```python
from build123d import *

# Parameters (mm, degrees)
VARREDURA_FINO1_PROFILE_R   = 6
VARREDURA_FINO1_PROFILE_R_2 = 5
RESSALTO_EXTRUS_O1_DEPTH    = 1


with BuildPart() as part:
    # Varredura-Fino1: sweep along a path in Esbo_o1
    with BuildLine(Plane.XY) as varredura_fino1_path:
        Line((0, -13.453624047), (-6.689647316, -7.432941462))
        ThreePointArc((-6.689647316, -7.432941462), (-9.74420246, 2.247335849), (-2.758518872, 9.612001541))
        Line((-2.758518872, 9.612001541), (13.460564792, 14.266666669))
    # Varredura-Fino1 profile (on start of the path) → Varredura-Fino1 (sweep)
    with BuildSketch(Plane(origin=(0, -13.453624047, 0), x_dir=(-0.6689647316224496, -0.7432941462471664, 0), z_dir=(-0.7432941462471664, 0.6689647316224496, 0))):
        Circle(VARREDURA_FINO1_PROFILE_R)
        Circle(VARREDURA_FINO1_PROFILE_R_2, mode=Mode.SUBTRACT)
    sweep(path=varredura_fino1_path.line)

    # Esbo_o19 → Ressalto-extrus_o1 (add)
    with BuildSketch(Plane(origin=(0, 0, -6), x_dir=(-1, 0, 0), z_dir=(0, 0, -1))):
        with BuildLine():
            Line((-13.046786961, 15.7084669), (-12.770935074, 16.669667054))
            Line((-12.770935074, 16.669667054), (-19.499336153, 18.600630265))
            ThreePointArc((-19.499336153, 18.600630265), (-22.591966256, 16.887259598), (-20.878595589, 13.794629494))
            Line((-20.878595589, 13.794629494), (-14.15019451, 11.863666283))
            Line((-14.15019451, 11.863666283), (-13.874342623, 12.824866438))
            Line((-13.874342623, 12.824866438), (-20.602743702, 14.755829648))
            ThreePointArc((-20.602743702, 14.755829648), (-21.630766102, 16.61140771), (-19.77518804, 17.639430111))
            Line((-19.77518804, 17.639430111), (-13.046786961, 15.7084669))
        make_face()
        with BuildLine():
            Line((-2.006894195, -11.223741608), (-2.675858926, -10.480447462))
            Line((-2.675858926, -10.480447462), (-7.87891795, -15.163200583))
            ThreePointArc((-7.87891795, -15.163200583), (-8.176235609, -20.812236095), (-2.527200097, -21.109553753))
            Line((-2.527200097, -21.109553753), (2.675858926, -16.426800632))
            Line((2.675858926, -16.426800632), (2.006894195, -15.683506486))
            Line((2.006894195, -15.683506486), (-3.196164829, -20.366259607))
            ThreePointArc((-3.196164829, -20.366259607), (-7.432941462, -20.143271363), (-7.209953219, -15.90649473))
            Line((-7.209953219, -15.90649473), (-2.006894195, -11.223741608))
        make_face()
    extrude(amount=-RESSALTO_EXTRUS_O1_DEPTH)


solid = part.part
```
Input: part model. Units: mm. Frame: model coordinates. A direction names the side the tool comes from. Coordinates: 2 decimals unless noted, no trailing zeros. Loops run counter-clockwise (first coordinate to the right, second up) from the corner with the lowest first, then second, coordinate; pieces in that order, holes last. Notation, with made-up numbers: (19.5, -16.5) - (35.5, -16.5) arc R15 cw to (35.5, -10.5) - close; hole circle Ø3 at (-23.5, 75). An arc over 180 degrees is marked (long way). Answer in a Markdown table with one row per item.
(1) Pin query (flat end, axial travel): P1, Ø4, axis at x = 4, z = -4, coming from the +Y side; P2, Ø5, axis at y = -8, z = -4, coming from the +X side; P3, Ø3.5, axis at x = 17.5, y = 14, coming from the +Z side. Return the tip coordinate at first contact, or that it passes through.
Model answer:
| item | result |
|---|---|
| P1 | stops at y = 17.62 |
| P2 | stops at x = 3.83 |
| P3 | stops at z = -5 |
(2) Mould query, pull axis Y, two halves, no side actions, for faces 1 (the face through (-2.667, -9.595, -4.881)), 2 (the face through (7, -15, -6)), 3 (the face through (6.84, 7.17, 0.22)), 4 (the face through (-0.04, -18.8, -5.51)). Classes: pulls with the +Y half, pulls with the -Y half, needs draft (parallel to the pull), parting line crosses it, or undercut.
Model answer:
| item | result |
|---|---|
| face 1 | undercut |
| face 2 | needs draft |
| face 3 | undercut |
| face 4 | pulls with the -Y half |
(3) Set-up query: faces 5 (the face through (5.24, -12.79, -5.51)), 6 (the face through (19, 14, -6)), 7 (the face through (0.558, -17.992, -5.507)). Return all of +Z, -Z, +X, -X, +Y, -Y with unobstructed straight access to the full face (end or side cutting, diameter ignored); none if empty.
Model answer:
| item | result |
|---|---|
| face 5 | +Z, -Z, +X |
| face 6 | -Z, +X, -X, +Y, -Y |
| face 7 | +Z, -Z |
(4) Material intervals for L1, parallel to Y at x = -3, z = -1.5; L2, parallel to Y at x = -1, z = -2.75; L3, parallel to Y at x = 7.5, z = -3.5, sorted ascending. Write a range as from..to.
Model answer:
| item | result |
|---|---|
| L1 | y = -4.34..-2.93, 2.93..4.28, 14.5..15.59 |
| L2 | y = -6.94..-5.38, 4.57..5.77, 14.46..15.66 |
| L3 | y = 7.49..8.84, 16.27..17.63 |
(5) Cut plane D-D on z = -2. Output: boundary loops of the cut face in (x, y).
Model answer:
| item | result |
|---|---|
| outline | (-10.47, -11.64) - (-3.78, -17.66) - (-3.07, -16.86) - (-9.76, -10.84) arc R14.58 cw to (-4.02, 14.02) - (12.2, 18.67) - (11.9, 19.7) - (-4.32, 15.05) arc R15.66 ccw to start; (-3.62, -4.03) - (3.07, -10.05) - (3.78, -9.25) - (-2.91, -3.23) arc R4.34 cw to (-1.2, 4.17) - (15.02, 8.83) - (14.72, 9.86) - (-1.49, 5.21) arc R5.42 ccw to start |
(6) Cut plane B-B on z = 0.75. Output: boundary loops of the cut face in (x, y), plus the area to 3 significant figures.
Model answer:
| item | result |
|---|---|
| outline | (-10.67, -11.86) - (-3.98, -17.88) - (-3.31, -17.13) - (-10, -11.11) arc R14.94 cw to (-4.12, 14.36) - (12.1, 19.02) - (11.82, 19.99) - (-4.4, 15.33) arc R15.95 ccw to start; (-3.38, -3.76) - (3.31, -9.78) - (3.98, -9.03) - (-2.71, -3.01) arc R4.05 cw to (-1.12, 3.89) - (15.1, 8.54) - (14.82, 9.52) - (-1.39, 4.86) arc R5.06 ccw to start |
| area | 95.2 mm² |
(7) Cut plane A-A on x = 18. Output: boundary loops of the cut face in (y, z), plus the area to 3 significant figures.
Model answer:
| item | result |
|---|---|
| outline | (12.97, -6) - (14.01, -6) - (14.01, -5) - (12.97, -5) - close; (17.13, -6) - (18.17, -6) - (18.17, -5) - (17.13, -5) - close |
| area | 2.08 mm² |
